Check sheet for the modelled part. Datum: model origin and axes. Units: mm. A direction names the side the tool comes from. Give positions to 0.01 mm unless a question says otherwise; leave off trailing zeros. Order: outer loops, then holes, each group sorted by start corner. A loop starts at its lowest first (then second) coordinate and runs counter-clockwise, first axis right, second up. Notation, with made-up numbers: (-20.75, 37.5) -> (38.25, 37.5) arc R11 ccw to (38.25, 55.5) -> close; hole circle Ø2 at (74, 2.5). An arc over 180 degrees is marked (long way). Write each question's results on one line, items separated by ' | '.
Autodesk Inventor part; units mm, degrees
ref_plane "YZ Plane" through (0, 0, 0) normal (1, 0, 0) x (0, 1, 0)
ref_plane "XZ Plane" through (0, 0, 0) normal (0, 1, 0) x (-1, 0, 0)
ref_plane "XY Plane" through (0, 0, 0) normal (0, 0, 1) x (1, 0, 0)
sketch "Sketch1" plane through (0, 0, 0) normal (1, 0, 0) x (0, 1, 0)
  line L0 (2.5981, 0) -> (1.299, -2.25)
  line L1 (1.299, -2.25) -> (-1.299, -2.25)
  line L2 (-1.299, -2.25) -> (-2.5981, 0)
  line L3 (-2.5981, 0) -> (-1.299, 2.25)
  line L4 (-1.299, 2.25) -> (1.299, 2.25)
  line L5 (1.299, 2.25) -> (2.5981, 0)
  point P0 (0, 0)
  point P1 (0, 0)
  dimension "d0" = 4.5
extrude "Extrusion1" add sketch "Sketch1" along normal blind 5
sketch "Sketch2" plane through (5, 0, 0) normal (1, 0, 0) x (0, 0, -1)
  circle A0 centre (0, 0) radius 1.5
  dimension "d3" = 3
extrude "Extrusion2" add sketch "Sketch2" against normal blind 13.2
sketch "Sketch3" plane through (5, 0, 0) normal (1, 0, 0) x (0, 0, -1)
  point P0 (0, 0)
  point P1 (0, 0)
hole "Hole1" at (5, 0, 0) direction (-1, 0, 0) diameter 2.459 depth 4.5 tip angle 118
thread "Thread1"
chamfer "Chamfer1" distance 0.3 angle 45 1 edges at (-8.2, 0, 1.5)
sketch "Sketch4" plane through (0, 0, 0) normal (0, 1, 0) x (-1, 0, 0)
  line L0 (0, 2.25) -> (-1.7321, 5.25)
  line L1 (-1.7321, 5.25) -> (0, 5.25)
  line L2 (0, 5.25) -> (0, 2.25)
  line L3 (-3.2679, 5.25) -> (-5, 2.25)
  line L4 (-5, 2.25) -> (-5, 5.25)
  line L5 (-5, 5.25) -> (-3.2679, 5.25)
  line L6 (10.84, 0) -> (-7.64, 0)
  point P0 (0, 0)
  dimension "d19" = 30
  dimension "d20" = 3
revolve "Revolution1" cut sketch "Sketch4" angle 360 about axis through (-10, 0, 0) along (1, 0, 0)
properties part number "Befestigungsbolzen_M3x13-2_Provertha-531333T" material "Steel"
1. Access from +Z, -Z, +X, -X, +Y, -Y to the whole of each face (thin tool, end or side, straight path). Record for faces 4 (the conical face through (0.086, 1.194, -2.081)), 5 (the cylindrical face through (-3.89, 0.07, 1.5)).
Verdict:
face 4: -Z, -X, +Y | face 5: -X
2. Mould release check, pull along Z, two halves, no side actions. Record for faces 1 (the conical face through (4.914, -1.194, -2.081)), 2 (the conical face through (-0.11, 0.064, -0.204)), 3 (the flat face through (2.46, 1.94, 1.14)): +Z half, -Z half, draft (parallel to the pull), parting line (faces both ways), or undercut.
Verdict:
face 1: -Z half | face 2: undercut | face 3: +Z half
3. Gauge pin test, flat ends, axial feed: pin 1 Ø1.5 at (x, z) = (-5, 1) entering from -Y; pin 2 Ø1.5 at (x, z) = (2, -0.5) entering from -Y; pin 3 Ø1 at (x, y) = (-4.5, 0.5) entering from -Z. Record the tip position at first contact, or that the pin passes through.
Verdict:
pin 1: stops at y = -1.48 | pin 2: stops at y = -2.6 | pin 3: stops at z = -1.5
4. Section check A-A on x = -3. Record the cut outline in (y, z), then the cut area to 3 significant figures.
Verdict:
outline: circle Ø3 at (0, 0) | area: 7.07 mm^2
5. Material ranges on probe 1 along Z at (x, y) = (3.1, 0); probe 2 along X at (y, z) = (0.75, -2.1); probe 3 along Y at (x, z) = (2.5, -1.05), recorded low to high. Write a range as from..to.
Verdict:
probe 1: z = -2.25..-1.23, 1.23..2.25 | probe 2: x = 0..5 | probe 3: y = -1.99..-0.64, 0.64..1.99
